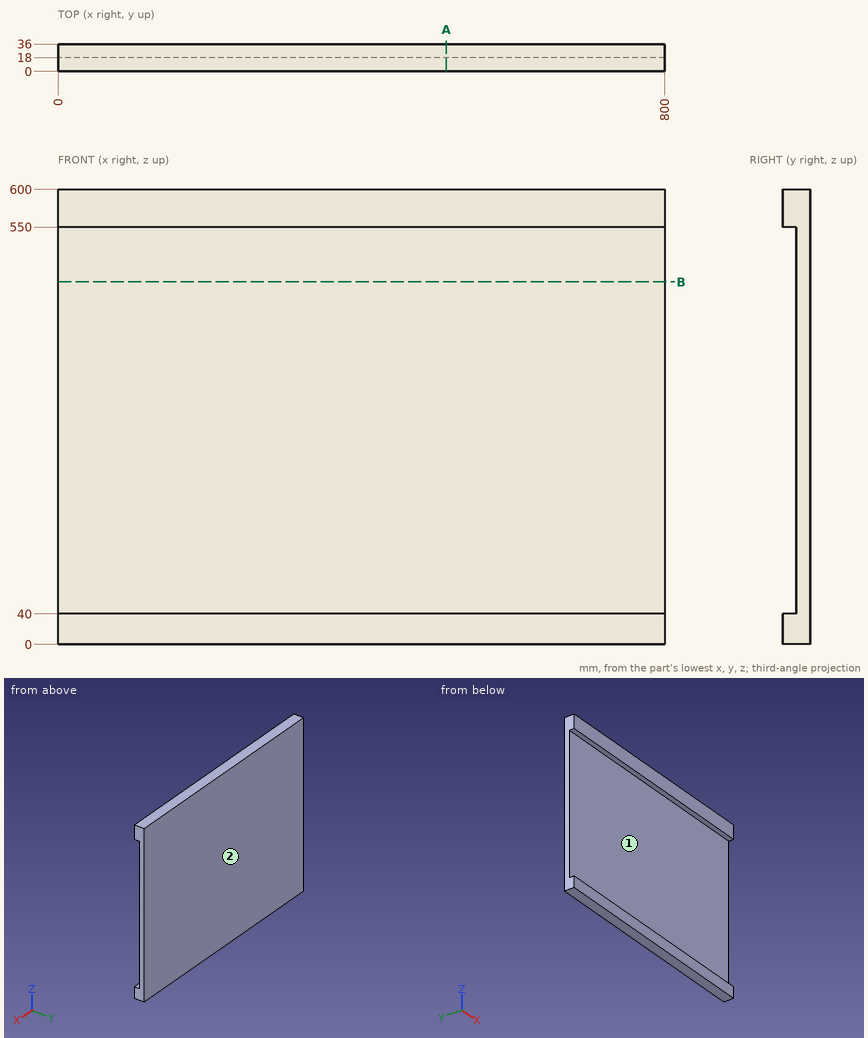
The drawing under review shows one solid part. Ordinate dimensions are in mm from its lowest x, y, z. Round coordinates to 2 decimals unless told otherwise and drop trailing zeros. Loops run counter-clockwise (first coordinate to the right, second up) from the corner with the lowest first, then second, coordinate; pieces in that order, holes last.
Item 1: Mouldability with a two-part tool opening along Z and no side actions: class the marked faces 1 and 2 as released by +Z, released by -Z, zero draft, split by the parting line, or undercut.
Determined:
face 1: undercut
face 2: zero draft
Item 2: For line 1 (Z direction, x = 213, y = 17.5); line 2 (Y direction, x = 692, z = 115.5), list the stretches that pass through material, from the lowest coordinate up.
Determined:
line 1: z = 0 to 40, 550 to 600
line 2: y = 18 to 36
Item 3: Clearance check with flat-ended pins moving along their axes: pin 1 Ø6 at (x, z) = (261.5, 400) entering from -Y; pin 2 Ø3 at (x, y) = (582, 12.5) entering from -Z. State where each tip first meets the part, or that it passes through.
Determined:
pin 1: stops at y = 18
pin 2: stops at z = 0
Item 4: Take a section at A-A (x = 512). Write out the cut boundary in (y, z), then the cut area to 3 significant figures.
Determined:
outline: (0, 0) - (36, 0) - (36, 600) - (0, 600) - (0, 550) - (18, 550) - (18, 40) - (0, 40) - close
area: 12,400 mm2
Item 5: Take a section at B-B (z = 478). Write out the cut boundary in (x, y), then the cut area to 3 significant figures.
Determined:
outline: (0, 18) - (800, 18) - (800, 36) - (0, 36) - close
area: 14,400 mm2
